```python
from build123d import *

# Parameters (mm, degrees)
SKETCH1_W                   = 50.8
SKETCH1_H                   = 85.09
BOSS_EXTRUDE1_DEPTH         = 35.7124
CUT_EXTRUDE1_REACH          = 88.93
SKETCH2_W                   = 31.749988824
SKETCH2_H                   = 31.04515
SKETCH4_W                   = 31.749988824
SKETCH4_H                   = 14.224
CUT_EXTRUDE2_DEPTH          = 87.929506383
CUT_EXTRUDE3_REACH          = 88.93
SKETCH5_W                   = 19.05
SKETCH5_H                   = 9.525
CUT_EXTRUDE4_START          = -71.4248
SKETCH6_W                   = 6.35
SKETCH6_H                   = 31.81985
CUT_EXTRUDE4_DEPTH          = 71.4248
F_10_CLEARANCE_HOLE1_D      = 4.9784
F_3_8_CLEARANCE_HOLE1_D     = 9.8044
F_3_8_CLEARANCE_HOLE1_DEPTH = 6.35
F_3_8_16_TAPPED_HOLE1_D     = 7.9375
F_3_8_16_TAPPED_HOLE1_DEPTH = 6.35
FILLET1_R                   = 3.175


with BuildPart() as part:
    # Sketch1 → Boss-Extrude1 (new, symmetric)
    with BuildSketch(Plane.XY):
        Rectangle(SKETCH1_W, SKETCH1_H)
    extrude(amount=BOSS_EXTRUDE1_DEPTH, both=True)

    # Sketch2 → Cut-Extrude1 (cut, up to next)
    with BuildSketch(Plane.XY.offset(35.7124), mode=Mode.PRIVATE) as cut_extrude1_sk1:
        with Locations((9.525005588, -4.797425)):
            Rectangle(SKETCH2_W, SKETCH2_H)
    cut_extrude1_tool1 = extrude(cut_extrude1_sk1.sketch, amount=-CUT_EXTRUDE1_REACH, mode=Mode.PRIVATE) & part.part
    add(cut_extrude1_tool1.solids().sort_by_distance((9.525006, -4.797425, 35.7124))[0], mode=Mode.SUBTRACT)

    # Sketch4 → Cut-Extrude2 (cut, through all)
    with BuildSketch(Plane.XY.offset(35.7124)):
        with Locations((9.525005588, 24.18715)):
            Rectangle(SKETCH4_W, SKETCH4_H)
    extrude(amount=-CUT_EXTRUDE2_DEPTH, mode=Mode.SUBTRACT)

    # Sketch5 → Cut-Extrude3 (cut, up to next)
    with BuildSketch(Plane.XY.offset(35.7124), mode=Mode.PRIVATE) as cut_extrude3_sk1:
        with Locations((15.875, -31.4325)):
            Rectangle(SKETCH5_W, SKETCH5_H)
    cut_extrude3_tool1 = extrude(cut_extrude3_sk1.sketch, amount=-CUT_EXTRUDE3_REACH, mode=Mode.PRIVATE) & part.part
    add(cut_extrude3_tool1.solids().sort_by_distance((15.875, -31.4325, 35.7124))[0], mode=Mode.SUBTRACT)

    # Sketch6 → Cut-Extrude4 (cut)
    with BuildSketch(Plane.XY.offset(35.7124).offset(CUT_EXTRUDE4_START)):
        with Locations((22.225, 26.635075)):
            Rectangle(SKETCH6_W, SKETCH6_H)
    extrude(amount=CUT_EXTRUDE4_DEPTH, mode=Mode.SUBTRACT)

    # #10 Clearance Hole1 (through all)
    with Locations(Plane.ZY.offset(25.4)):
        with Locations((0, 24.13)):
            Hole(F_10_CLEARANCE_HOLE1_D / 2)

    # 3/8 Clearance Hole1
    with Locations(Plane(origin=(0, -42.545, 0), x_dir=(-1, 0, 0), z_dir=(0, -1, 0))):
        with Locations((-15.875, -19.05), (-15.875, 19.05)):
            Hole(F_3_8_CLEARANCE_HOLE1_D / 2, depth=F_3_8_CLEARANCE_HOLE1_DEPTH)

    # 3/8-16 Tapped Hole1
    with Locations(Plane(origin=(0, -20.32, 0), x_dir=(1, 0, 0), z_dir=(0, 1, 0))):
        with Locations((15.875, -19.05), (15.875, 19.05)):
            Hole(F_3_8_16_TAPPED_HOLE1_D / 2, depth=F_3_8_16_TAPPED_HOLE1_DEPTH)

    # Fillet1
    fillet1_edges = [part.edges().sort_by_distance(p)[0] for p in [
        (-6.349988824, -20.32, 0),
        (-6.349988824, 10.72515, 0),
    ]]
    fillet(fillet1_edges, radius=FILLET1_R)


solid = part.part
```
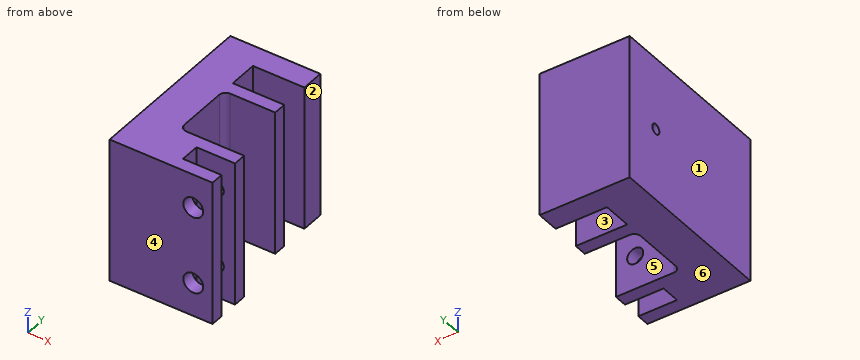
Source: CAD feature listing. Evaluate the final solid. Frame: model axes, mm. Face numbers are marked on the shaded views. A direction names the side the tool comes from. Give positions to 0.01 mm unless a question says otherwise; leave off trailing zeros. Loops run counter-clockwise (first coordinate to the right, second up) from the corner with the lowest first, then second, coordinate; pieces in that order, holes last. Notation, with made-up numbers: (0, -21.5) -> (35, -21.5) arc R22 cw to (35, -3.5) -> close; hole circle Ø4 at (-34, -22). An arc over 180 degrees is marked (long way). Use a Markdown table: item, result. Add a question column.
(1) Ray query, line 1 (Y direction, x = 9, z = 4.5) (3 decimals); line 2 (Y direction, x = -6, z = -3) (3 decimals); line 3 (Y direction, x = 21, z = 0) (3 decimals). Return the intervals inside material, ascending.
(2) Section query A-A (y = 24.13). Output: boundary loops of the cut face in (x, z), then the cut area to 3 significant figures.
(3) Access query for the marked faces 1, 2 and 3. Directions: +Z, -Z, +X, -X, +Y, -Y. A direction counts if a zero-diameter tool reaches every point of the face in a straight line with its end or side. Return the directions, or none.
(4) Section query D-D (z = 10). Output: boundary loops of the cut face in (x, y) (3 decimals), then the cut area to 3 significant figures.
(5) Section query C-C (z = 19.05). Output: boundary loops of the cut face in (x, y) (3 decimals), then the cut area to 3 significant figures.
(6) Pull-direction query (Y, two-part tool) for the marked faces 4, 5 and 6; classes: +Y half, -Y half, draft (parallel to the pull), parting line (faces both ways), or undercut.
(7) First-contact query: pin 1 Ø1.5 at (x, z) = (17, -23) entering from -Y; pin 2 Ø7 at (x, z) = (15.875, -19.05) entering from -Y; pin 3 Ø6 at (y, z) = (-3, -24.5) entering from +X; pin 4 Ø12 at (x, y) = (-5.5, 25.5) entering from -Z. Flat tips, straight axial feed; report the tip coordinate or a pass-through.
(8) Section query B-B (x = 2). Output: boundary loops of the cut face in (y, z) (3 decimals).
Checked values:
| question | item | result |
|---|---|---|
| 1 | line 1 | -42.545 to -36.195, -26.67 to -20.32, 10.725 to 17.075, 31.299 to 42.545 |
| 1 | line 2 | -42.545 to -18.594, 8.999 to 17.075, 31.299 to 42.545 |
| 1 | line 3 | -42.545 to -36.195, -26.67 to -20.32 |
| 2 | outline | (-25.4, -35.71) -> (-6.35, -35.71) -> (-6.35, -2.49) -> (-25.4, -2.49) -> close; (-25.4, 2.49) -> (-6.35, 2.49) -> (-6.35, 35.71) -> (-25.4, 35.71) -> close |
| 2 | area | 1,270 mm^2 |
| 3 | face 1 | +Z, -Z, -X, +Y, -Y |
| 3 | face 2 | +Z, -Z, +X, +Y |
| 3 | face 3 | +Z, -Z, +X |
| 4 | outline | (-25.4, -42.545) -> (25.4, -42.545) -> (25.4, -36.195) -> (6.35, -36.195) -> (6.35, -26.67) -> (25.4, -26.67) -> (25.4, -20.32) -> (-3.175, -20.32) arc R3.175 cw to (-6.35, -17.145) -> (-6.35, 7.55) arc R3.175 cw to (-3.175, 10.725) -> (19.05, 10.725) -> (19.05, 17.075) -> (-6.35, 17.075) -> (-6.35, 31.299) -> (19.05, 31.299) -> (19.05, 42.545) -> (-25.4, 42.545) -> close |
| 4 | area | 2,600 mm^2 |
| 5 | outline | (-25.4, -42.545) -> (10.973, -42.545) -> (10.973, -36.195) -> (6.35, -36.195) -> (6.35, -26.67) -> (11.906, -26.67) -> (11.906, -20.32) -> (-3.175, -20.32) arc R3.175 cw to (-6.35, -17.145) -> (-6.35, 7.55) arc R3.175 cw to (-3.175, 10.725) -> (19.05, 10.725) -> (19.05, 17.075) -> (-6.35, 17.075) -> (-6.35, 31.299) -> (19.05, 31.299) -> (19.05, 42.545) -> (-25.4, 42.545) -> close; (19.844, -26.67) -> (25.4, -26.67) -> (25.4, -20.32) -> (19.844, -20.32) -> close; (20.777, -42.545) -> (25.4, -42.545) -> (25.4, -36.195) -> (20.777, -36.195) -> close |
| 5 | area | 2,480 mm^2 |
| 6 | face 4 | -Y half |
| 6 | face 5 | undercut |
| 6 | face 6 | draft |
| 7 | pin 1 | y = -26.67 |
| 7 | pin 2 | y = 10.73 |
| 7 | pin 3 | x = -6.35 |
| 7 | pin 4 | z = -35.71 |
| 8 | outline | (-42.545, -35.712) -> (-20.32, -35.712) -> (-20.32, 35.712) -> (-42.545, 35.712) -> close; (10.725, -35.712) -> (17.075, -35.712) -> (17.075, 35.712) -> (10.725, 35.712) -> close; (31.299, -35.712) -> (42.545, -35.712) -> (42.545, 35.712) -> (31.299, 35.712) -> close |
